Study the drawing (mm; zero at the part's minimum x, y, z) and answer. A direction names the side the tool comes from. Coordinates: 2 decimals unless noted, no trailing zeros. Order: outer loops, then holes, each group sorted by start corner. A loop starts at its lowest first (then second) coordinate and runs counter-clockwise, first axis right, second up. Notation, with made-up numbers: (-24.75, 79.25) - (31.25, 79.25) arc R31 cw to (31.25, 108.25) - close; hole circle Ø2 at (13.5, 34.25). An arc over 180 degrees is marked (long way). Write item = value, one per line.
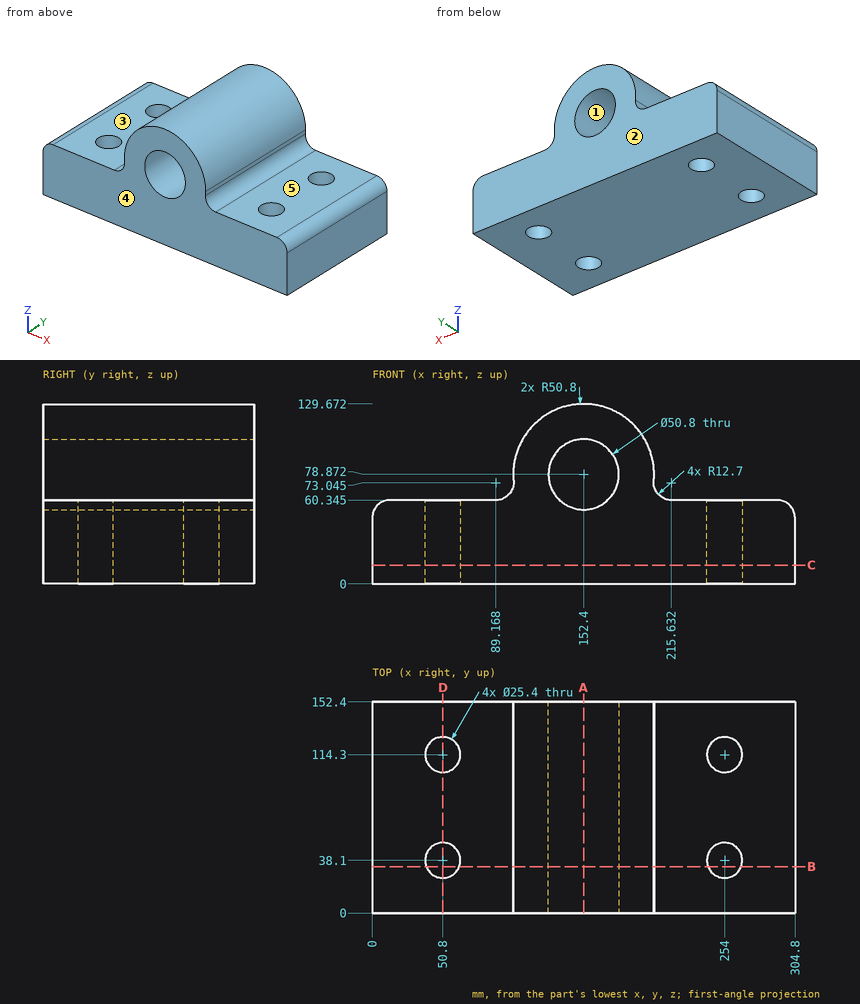
1) For the marked faces 4 and 5, determine the directions among +Z, -Z, +X, -X, +Y, -Y from which every point of the face is accessible in a straight line to the end or side of a thin tool.
Returned:
face_4 = +Z, -Z, +X, -X, -Y
face_5 = +Z, +X, +Y, -Y
2) Flat-ended cylindrical pins translate along their axes: pin 1 Ø15 at (x, y) = (254, 114.3) entering from -Z; pin 2 Ø1.5 at (x, y) = (63, 107) entering from -Z; pin 3 Ø2 at (y, z) = (63, 97.5) entering from -X; pin 4 Ø6 at (x, y) = (253.5, 125.5) entering from +Z (3 decimals). Find the tip coordinate at first contact, or state that the pin passes through.
Returned:
pin_1 = through
pin_2 = 0
pin_3 = 104.76
pin_4 = 60.345
3) The part is cut by section D-D (x = 50.8). Determine the outline of the cut face in (y, z) (1 decimal), and give its area (3 significant figures).
Returned:
outline = (0, 0) - (25.4, 0) - (25.4, 60.3) - (0, 60.3) - close; (50.8, 0) - (101.6, 0) - (101.6, 60.3) - (50.8, 60.3) - close; (127, 0) - (152.4, 0) - (152.4, 60.3) - (127, 60.3) - close
area = 6,130 mm^2
4) The part is cut by section A-A (x = 152.4). Determine the outline of the cut face in (y, z).
Returned:
outline = (0, 0) - (152.4, 0) - (152.4, 53.47) - (0, 53.47) - close; (0, 104.27) - (152.4, 104.27) - (152.4, 129.67) - (0, 129.67) - close
5) The part is cut by section C-C (z = 13.5). Determine the outline of the cut face in (x, y), and give its area (3 significant figures).
Returned:
outline = (0, 0) - (304.8, 0) - (304.8, 152.4) - (0, 152.4) - close; hole circle Ø25.4 at (50.8, 38.1); hole circle Ø25.4 at (50.8, 114.3); hole circle Ø25.4 at (254, 38.1); hole circle Ø25.4 at (254, 114.3)
area = 44,400 mm^2
6) The part is cut by section B-B (y = 33.5). Determine the outline of the cut face in (x, z) (1 decimal), and give its area (3 significant figures).
Returned:
outline = (0, 0) - (39, 0) - (39, 60.3) - (12.7, 60.3) arc R12.7 ccw to (0, 47.6) - close; (62.6, 0) - (242.2, 0) - (242.2, 60.3) - (215.6, 60.3) arc R12.7 cw to (203, 74.2) arc R50.8 ccw to (203.2, 78.9) arc R50.8 ccw (long way) to (101.8, 74.2) arc R12.7 cw to (89.2, 60.3) - (62.6, 60.3) - close; (265.8, 0) - (304.8, 0) - (304.8, 47.6) arc R12.7 ccw to (292.1, 60.3) - (265.8, 60.3) - close; hole circle Ø50.8 at (152.4, 78.9)
area = 19,400 mm^2
7) Determine the mould class of the marked faces 1, 2 and 3 for opening direction Z: pulls with the +Z half, pulls with the -Z half, needs draft (parallel to the pull), parting line crosses it, or undercut.
Returned:
face_1 = undercut
face_2 = needs draft
face_3 = pulls with the +Z half
8) Straight lines are drawn through the part: line 1 along Y through (x, z) = (50, 33) (1 decimal); line 2 along X through (y, z) = (121, 10.5); line 3 along Z through (x, y) = (154, 106). For each, find the intervals that lie inside material, in ascending order. Write a range as from..to.
Returned:
line_1 = 0..25.4, 50.8..101.6, 127..152.4
line_2 = 0..40.01, 61.59..243.21, 264.79..304.8
line_3 = 0..53.52, 104.22..129.65
